Geometry check sheet. Reference: the model listing, model coordinates, mm. A direction names the side the tool comes from. Round coordinates to 2 decimals unless told otherwise and drop trailing zeros. Order: outer loops, then holes, each group sorted by start corner. A loop starts at its lowest first (then second) coordinate and runs counter-clockwise, first axis right, second up. Notation, with made-up numbers: M -4,-13 L 34,-13 A17 ccw 34,16 Z; hole C 64,-15 d7. An arc over 180 degrees is marked long. Return JSON: item names as keys, results as strings. Group by question number.
```python
from build123d import *

# Parameters (mm, degrees)
F0_R      = 0.8
F0_R_2    = 3.2
F1_DEPTH  = 6
F3_DEPTH  = 6
F4_W      = 4.4655336533
F4_H      = 0.3993565915
F4_W_2    = 0.3993565915
F4_H_2    = 4.4655336533
F5_DEPTH  = 4.5
F6_R      = 0.7
F7_DEPTH  = 5
F8_R      = 0.7
F9_DEPTH  = 1
F0_R_3    = 1
F10_DEPTH = 10
F11_DEPTH = 10


with BuildPart() as f1:
    # F0 (on Front) → F1 (new body)
    with BuildSketch(Plane.XZ):
        with BuildLine():
            Line((-7, -4.5), (7, -4.5))
            ThreePointArc((7, -4.5), (10.1819805153, -3.1819805153), (11.5, 0))
            ThreePointArc((11.5, 0), (10.1819805153, 3.1819805153), (7, 4.5))
            Line((7, 4.5), (-7, 4.5))
            ThreePointArc((-7, 4.5), (-10.1819805153, 3.1819805153), (-11.5, 0))
            ThreePointArc((-11.5, 0), (-10.1819805153, -3.1819805153), (-7, -4.5))
        make_face()
        with Locations((-9, 0)):
            Circle(F0_R, mode=Mode.SUBTRACT)
        Circle(F0_R_2, mode=Mode.SUBTRACT)
        with Locations((9, 0)):
            Circle(F0_R, mode=Mode.SUBTRACT)
    extrude(amount=-F1_DEPTH)

    # F2 (on face) → F3 (join)
    with BuildSketch(Plane(origin=(0, 6, 0), x_dir=(-1, 0, 0), z_dir=(0, 1, 0))):
        with BuildLine():
            Line((7, 4.5), (-2.3691008836, 4.5))
            ThreePointArc((-2.3691008836, 4.5), (-5.1975280083, 3.3284271247), (-6.3691008836, 0.5))
            Line((-6.3691008836, 0.5), (-6.3691008836, -0.5))
            ThreePointArc((-6.3691008836, -0.5), (-5.1975280083, -3.3284271247), (-2.3691008836, -4.5))
            Line((-2.3691008836, -4.5), (7, -4.5))
            Line((7, -4.5), (7, 4.5))
        make_face()
    extrude(amount=F3_DEPTH)

    # F4 (on face) → F5 (join)
    with BuildSketch(Plane(origin=(0, 12, 0), x_dir=(-1, 0, 0), z_dir=(0, 1, 0))):
        with Locations((1.0412741685, 3.2637477852)):
            Rectangle(F4_W, F4_H)
        with Locations((1.0412741685, 0.8087011712)):
            Rectangle(F4_W, F4_H)
        with Locations((5.7582546142, -0.0916777644)):
            Rectangle(F4_W_2, F4_H_2)
    extrude(amount=F5_DEPTH)

    # F6 (on face) → F7 (cut)
    with BuildSketch(Plane.XY.offset(3.463426081)):
        with Locations((-1.0412741685, 14.6806975827)):
            Circle(F6_R)
    extrude(amount=-F7_DEPTH, mode=Mode.SUBTRACT)

    # F8 (on face) → F9 (cut)
    with BuildSketch(Plane.YZ.offset(-5.5585763184)):
        with Locations((14.6806975827, -0.0916777644)):
            Circle(F8_R)
    extrude(amount=-F9_DEPTH, mode=Mode.SUBTRACT)

    # F0 (on Front) → F10 (cut)
    with BuildSketch(Plane.XZ):
        Circle(F0_R_2)
        Circle(F0_R_3, mode=Mode.SUBTRACT)
    extrude(amount=-F10_DEPTH, mode=Mode.SUBTRACT)

    # F0 (on Front) → F11 (join)
    with BuildSketch(Plane.XZ):
        Circle(F0_R_3)
    extrude(amount=-F11_DEPTH)


solid = f1.part
```
Q1. Material ranges on line 1 along Z through (x, y) = (0, 3.25); line 2 along Z through (x, y) = (-0.5, 8.5); line 3 along Y through (x, z) = (10.5, -1), recorded low to high.
Q2. Depth check by flat-ended pin: pin 1 Ø2 at (x, y) = (0, 14) entering from -Z; pin 2 Ø0.8 at (y, z) = (8, 0) entering from +X; pin 3 Ø2 at (y, z) = (15, 1) entering from -X. Enter the tip coordinate at first touch or a pass-through.
Q3. Section check B-B on x = 9. Record the cut outline in (y, z).
Q4. Section check C-C on y = 15. Record the cut outline in (x, z), plus the area to 3 significant figures.
Q5. Set-up check for faces 1 (the face through (-1, 13.7, 1.008)), 2 (the face through (5.228, 8.958, -3.297)), 3 (the face through (5.166, 8.958, 3.359)): record each of +Z, -Z, +X, -X, +Y, -Y from which the full face is reachable in a straight line by a thin tool's end or side.
Q6. Section check D-D on x = 0. Record the cut outline in (y, z), plus the area to 3 significant figures.
Q7. Section check A-A on y = 5.5. Record the cut outline in (x, z).
Q8. Release check for a two-part mould opening along X. For faces 4 (the face through (8.41, 2.96, 0.54)), 5 (the face through (-7, 9, 0)), 6 (the face through (-5.755, 14.125, -0.518)), 7 (the face through (6.369, 9, 0)) record: +X half, -X half, draft (parallel to the pull), parting line (faces both ways), or undercut.
Geometry check:
{
 "1": {"line 1": "z = -4.5 to -3.2, -1 to 1, 3.2 to 4.5", "line 2": "z = -4.5 to -3.16, -0.87 to 0.87, 3.16 to 4.5", "line 3": "y = 0 to 6"},
 "2": {"pin 1": "stops at z = 0.61", "pin 2": "stops at x = 6.37", "pin 3": "stops at x = -5.96"},
 "3": {"outline": "M 0,-4.03 L 6,-4.03 L 6,-0.8 L 0,-0.8 Z; M 0,0.8 L 6,0.8 L 6,4.03 L 0,4.03 Z"},
 "4": {"outline": "M -5.96,-2.32 L -5.56,-2.32 L -5.56,-0.71 L -5.96,-0.71 Z; M -5.96,0.53 L -5.56,0.53 L -5.56,2.14 L -5.96,2.14 Z; M -3.27,0.61 L -1.66,0.61 L -1.66,1.01 L -3.27,1.01 Z; M -3.27,3.06 L -1.66,3.06 L -1.66,3.46 L -3.27,3.46 Z; M -0.42,0.61 L 1.19,0.61 L 1.19,1.01 L -0.42,1.01 Z; M -0.42,3.06 L 1.19,3.06 L 1.19,3.46 L -0.42,3.46 Z", "area": "3.86 mm^2"},
 "5": {"face 1": "+X, +Y", "face 2": "-Z, +X, +Y", "face 3": "+Z, +X, +Y"},
 "6": {"outline": "M 0,-4.5 L 12,-4.5 L 12,0.61 L 16.5,0.61 L 16.5,1.01 L 12,1.01 L 12,3.06 L 16.5,3.06 L 16.5,3.46 L 12,3.46 L 12,4.5 L 0,4.5 L 0,3.2 L 10,3.2 L 10,1 L 0,1 L 0,-1 L 10,-1 L 10,-3.2 L 0,-3.2 Z", "area": "67.6 mm^2"},
 "7": {"outline": "M -7,-4.5 L 7,-4.5 A4.5 ccw 7,4.5 L -7,4.5 A4.5 ccw Z; C 0,0 d2; hole C -9,0 d1.6; hole C 0,0 d6.4; hole C 9,0 d1.6"},
 "8": {"face 4": "undercut", "face 5": "-X half", "face 6": "draft", "face 7": "+X half"}
}
